Work out the finished part from the listing and answer in its coordinate system (mm). A direction names the side the tool comes from. Coordinates: 2 decimals unless noted, no trailing zeros. Order: outer loops, then holes, each group sorted by start corner. A loop starts at its lowest first (then second) coordinate and runs counter-clockwise, first axis right, second up. Notation, with made-up numbers: M 63.25,78 L 88.25,78 A20 cw 88.25,89 Z; hole C -27,59.25 d9. An arc over 180 degrees is marked long. Use a Markdown table: item, result. Add a question column.
from build123d import *

# Parameters (mm, degrees)
BOSS_EXTRUDE1_DEPTH = 5
SKETCH3_W           = 40
SKETCH3_H           = 5
BOSS_EXTRUDE2_DEPTH = 80
SKETCH4_R           = 2.5
CUT_EXTRUDE1_DEPTH  = 10
CUT_EXTRUDE2_DEPTH  = 10


with BuildPart() as part:
    # Sketch2 → Boss-Extrude1 (new body)
    with BuildSketch(Plane.XY):
        with BuildLine():
            Line((20, 0), (20, -25))
            Line((20, -25), (-20, -25))
            Line((-20, -25), (-20, 0))
            ThreePointArc((-20, 0), (0, 20), (20, 0))
        make_face()
        with BuildLine():
            Line((-15.5, 2.95), (15.5, 2.95))
            ThreePointArc((15.5, 2.95), (18.45, 0), (15.5, -2.95))
            Line((15.5, -2.95), (-15.5, -2.95))
            ThreePointArc((-15.5, -2.95), (-18.45, 0), (-15.5, 2.95))
        make_face(mode=Mode.SUBTRACT)
    extrude(amount=BOSS_EXTRUDE1_DEPTH)

    # Sketch3 → Boss-Extrude2 (add)
    with BuildSketch(Plane.XY.offset(5)):
        with Locations((0, -22.5)):
            Rectangle(SKETCH3_W, SKETCH3_H)
    extrude(amount=BOSS_EXTRUDE2_DEPTH)

    # Sketch4 → Cut-Extrude1 (cut)
    with BuildSketch(Plane(origin=(0, -20, 0), x_dir=(1, 0, 0), z_dir=(0, 1, 0))):
        with Locations((-15, -10)):
            Circle(SKETCH4_R)
        with Locations((15, -10)):
            Circle(SKETCH4_R)
        with Locations((15, -80)):
            Circle(SKETCH4_R)
        with Locations((-15, -80)):
            Circle(SKETCH4_R)
        with Locations((-15, -45)):
            Circle(SKETCH4_R)
        with Locations((15, -45)):
            Circle(SKETCH4_R)
    extrude(amount=-CUT_EXTRUDE1_DEPTH, mode=Mode.SUBTRACT)

    # Sketch5 → Cut-Extrude2 (cut)
    with BuildSketch(Plane.XY.offset(5)):
        with BuildLine():
            Line((6.5, 7), (6.5, -7))
            ThreePointArc((6.5, -7), (0, -13.5), (-6.5, -7))
            Line((-6.5, -7), (-6.5, 7))
            ThreePointArc((-6.5, 7), (0, 13.5), (6.5, 7))
        make_face()
    extrude(amount=-CUT_EXTRUDE2_DEPTH, mode=Mode.SUBTRACT)


solid = part.part
(1) Straight lines are drawn through the part: line 1 (X direction, y = -22, z = 80); line 2 (Z direction, x = 15, y = -23.6); line 3 (Y direction, x = 4.5, z = 29.5). For each, find the intervals that lie inside material, in ascending order.
(2) A cutting plane is placed at A-A on z = 80. Write down the section's boundary in (x, y).
(3) A cutting plane is placed at B-B on x = 0. Write down the section's boundary in (y, z).
(4) A cutting plane is placed at C-C on y = -2. Write down the section's boundary in (x, z), plus the area to 3 significant figures.
(5) The mould has two halves that part along Y. Classify faces 4 (the flat face through (0, -25, 42)), 5 (the flat face through (0, -22, 85)), 6 (the flat face through (6.5, 5, 3)): pulls with the +Y half, pulls with the -Y half, needs draft (parallel to the pull), parting line crosses it, or undercut.
(6) A cutting plane is placed at D-D on y = -8. Write down the section's boundary in (x, z).
(7) Given P1, Ø20, axis at x = 6, y = 3.5, coming from the +Z side; P2, Ø5, axis at x = 14, z = 70.5, coming from the +Y side; P3, Ø5.5, axis at x = -11, z = 2, coming from the +Y side, each flat-ended and moving along its own axis, determine where each tip first touches the part or whether it passes through.
(8) Which of the six approach directions +Z, -Z, +X, -X, +Y, -Y give full straight-line access (tool end or side, diameter ignored) to faces 1 (the flat face through (-4.2, -12.2, 0)), 2 (the flat face through (-9, -4, 5)), 3 (the flat face through (-6.5, -5, 3))?
From the geometry:
| question | item | result |
|---|---|---|
| 1 | line 1 | x = -20 to -17.5, -12.5 to 12.5, 17.5 to 20 |
| 1 | line 2 | z = 0 to 7.5, 12.5 to 42.5, 47.5 to 77.5, 82.5 to 85 |
| 1 | line 3 | y = -25 to -20 |
| 2 | outline | M -20,-25 L -17.5,-25 L -17.5,-20 L -20,-20 Z; M -12.5,-25 L 12.5,-25 L 12.5,-20 L -12.5,-20 Z; M 17.5,-25 L 20,-25 L 20,-20 L 17.5,-20 Z |
| 3 | outline | M -25,0 L -13.5,0 L -13.5,5 L -20,5 L -20,85 L -25,85 Z; M 13.5,0 L 20,0 L 20,5 L 13.5,5 Z |
| 4 | outline | M -20,0 L -17.67,0 L -17.67,5 L -20,5 Z; M 17.67,0 L 20,0 L 20,5 L 17.67,5 Z |
| 4 | area | 23.3 mm2 |
| 5 | face 4 | pulls with the -Y half |
| 5 | face 5 | needs draft |
| 5 | face 6 | undercut |
| 6 | outline | M -20,0 L -6.42,0 L -6.42,5 L -20,5 Z; M 6.42,0 L 20,0 L 20,5 L 6.42,5 Z |
| 7 | P1 | stops at z = 5 |
| 7 | P2 | stops at y = -20 |
| 7 | P3 | stops at y = 18.22 |
| 8 | face 1 | -Z, +X, -X, +Y, -Y |
| 8 | face 2 | +Z, +X, -X, +Y |
| 8 | face 3 | +Z, -Z |
